Part model, mm, in its own coordinate system. A direction names the side the tool comes from. Give positions to 0.01 mm unless a question says otherwise; leave off trailing zeros. Write each loop counter-clockwise with the first axis right and the second up, starting at its lowest first coordinate (ties: lowest second). Pieces come first, ordered by that corner, then holes. Notation, with made-up numbers: M 56,62.5 L 106,62.5 A25 cw 106,94.5 Z; hole C 74,81 d3. An arc over 180 degrees is marked long. Answer as CSV lines item,"result". Start each with the question number.
Item 1: 3-axis set-ups, long thin cutter, end or side, ignore diameter. For faces 1 (the flat face through (99, -45, 9.669)), 2 (the flat face through (0, -41.5, 94)), 3 (the flat face through (0, -48.5, 94)), 4 (the flat face through (-91.805, -45, -10)), 5 (the flat face through (-99, -45, 9.669)): which of +Z, -Z, +X, -X, +Y, -Y reach the whole face in a straight line?
Item 2: Band-saw the part on A-A, the plane y = -32.25. List the corners of the cut face in (x, z) (3 decimals).
Item 3: Two-plate mould, pull along Y, no slides. Class faces 6 (the flat face through (91.805, -45, -10)), 7 (the cylindrical face through (99.41, -39.554, -7.481)), 8 (the flat face through (-99, -60, -6)): +Y half, -Y half, draft (parallel to the pull), parting line (faces both ways), or undercut.
Item 4: Wall check: L1, parallel to X at y = -46.5, z = 1 (3 decimals); L2, parallel to Z at x = -95.5, y = -40.25; L3, parallel to Y at x = -62.5, z = 73.5. Give the ranges that are in metal, low to high. Write a range as from..to.
Item 5: Band-saw the part on C-C, the plane z = 32. List the corners of the cut face in (x, y), then the cut area to 3 significant figures.
Item 6: Band-saw the part on B-B, the plane z = 82.5. List the corners of the cut face in (x, y).
Item 7: Band-saw the part on D-D, the plane x = 0. List the corners of the cut face in (y, z) (3 decimals), then the cut area to 3 significant figures.
Item 8: Pin check, flat tips, straight feed: pin 1 (4 mm diameter, centred on x = -47.5, y = -42, fed in from +Z); pin 2 (13 mm diameter, centred on y = -42.93, z = -5.33, fed in from -X) (3 decimals); pin 3 (4.5 mm diameter, centred on x = -100.5, y = -40.5, fed in from +Z); pin 4 (8 mm diameter, centred on x = -42.5, y = -46.5, fed in from -Z). Stop position of each tip, or through.
from build123d import *

# Parameters (mm, degrees)
BOSS_EXTRUDE1_DEPTH      = 60
CUT_EXTRUDE19_DEPTH      = 171.881965709
CUT_EXTRUDE19_DEPTH_BACK = 171.881965709
SKETCH30_W               = 213.61
SKETCH30_H               = 30
SKETCH31_R               = 4
CUT_EXTRUDE20_DEPTH      = 243.881988062
CUT_EXTRUDE21_DEPTH      = 11.5
CUT_EXTRUDE22_START      = -11.5
CUT_EXTRUDE22_DEPTH      = 11.5


with BuildPart() as part:
    # Sketch1 → Boss-Extrude1 (new body)
    with BuildSketch(Plane(origin=(0, 0, 0), x_dir=(1, 0, 0), z_dir=(0, 1, 0))):
        with BuildLine():
            Line((106.805, -9.669202779), (98.330740578, -9.669202779))
            ThreePointArc((98.330740578, -9.669202779), (0, -98.805), (-98.330740578, -9.669202779))
            Line((-98.330740578, -9.669202779), (-106.805, -9.669202779))
            Line((-106.805, -9.669202779), (-106.805, 20.330797221))
            Line((-106.805, 20.330797221), (-91.805, 20.330797221))
            Line((-91.805, 20.330797221), (-91.805, 0))
            ThreePointArc((-91.805, 0), (0, -91.805), (91.805, 0))
            Line((91.805, 0), (91.805, 20.330797221))
            Line((91.805, 20.330797221), (106.805, 20.330797221))
            Line((106.805, 20.330797221), (106.805, -9.669202779))
        make_face()
    extrude(amount=-BOSS_EXTRUDE1_DEPTH)

    # Sketch30 → Cut-Extrude19 (cut, two sides: drawn at the far end of the back side and taken through both)
    with BuildSketch(Plane(origin=(0, 0, -20.330797221), x_dir=(-1, 0, 0), z_dir=(0, 0, -1)).offset(-CUT_EXTRUDE19_DEPTH_BACK)):
        with Locations((0, -15)):
            Rectangle(SKETCH30_W, SKETCH30_H)
    extrude(amount=CUT_EXTRUDE19_DEPTH + CUT_EXTRUDE19_DEPTH_BACK, mode=Mode.SUBTRACT)

    # Sketch31 → Cut-Extrude20 (cut, through all)
    with BuildSketch(Plane(origin=(106.805, 0, 0), x_dir=(0, 0, -1), z_dir=(1, 0, 0))):
        with Locations((5.330797221, -42.92674227)):
            Circle(SKETCH31_R)
    extrude(amount=-CUT_EXTRUDE20_DEPTH, mode=Mode.SUBTRACT)

    # Sketch32 → Cut-Extrude21 (cut)
    with BuildSketch(Plane(origin=(0, -30, 0), x_dir=(1, 0, 0), z_dir=(0, 1, 0))):
        with BuildLine():
            Line((98.330740578, -9.669202779), (-98.330740578, -9.669202779))
            ThreePointArc((-98.330740578, -9.669202779), (0, -98.805), (98.330740578, -9.669202779))
        make_face()
    extrude(amount=-CUT_EXTRUDE21_DEPTH, mode=Mode.SUBTRACT)

    # Sketch33 → Cut-Extrude22 (cut)
    with BuildSketch(Plane(origin=(0, -60, 0), x_dir=(-1, 0, 0), z_dir=(0, -1, 0)).offset(CUT_EXTRUDE22_START)):
        with BuildLine():
            Line((98.330740578, -9.669202779), (-98.330740578, -9.669202779))
            ThreePointArc((-98.330740578, -9.669202779), (0, -98.805), (98.330740578, -9.669202779))
        make_face()
    extrude(amount=CUT_EXTRUDE22_DEPTH, mode=Mode.SUBTRACT)


solid = part.part
Output:
1,face 1,"+Z, +X"
1,face 2,"+Z, +X, -X, +Y"
1,face 3,"+Z, +X, -X, -Y"
1,face 4,"-Z, +Y, -Y"
1,face 5,"+Z, -X"
2,outline,"M -106.805,-20.331 L -91.805,-20.331 L -91.805,0 A91.805 cw -91.294,9.669 L -106.805,9.669 Z; M 91.294,9.669 A91.805 cw 91.805,0 L 91.805,-20.331 L 106.805,-20.331 L 106.805,9.669 Z"
3,face 6,"draft"
3,face 7,"undercut"
3,face 8,"-Y half"
4,L1,"-106.805..-91.8, 91.8..106.805"
4,L2,"-20.33..-8.3, -2.36..9.67"
4,L3,"-48.5..-41.5"
5,outline,"M -93.48,-48.5 L -86.05,-48.5 L -86.05,-41.5 L -93.48,-41.5 Z; M 86.05,-48.5 L 93.48,-48.5 L 93.48,-41.5 L 86.05,-41.5 Z"
5,area,"104 mm²"
6,outline,"M -54.37,-48.5 L -40.27,-48.5 L -40.27,-41.5 L -54.37,-41.5 Z; M 40.27,-48.5 L 54.37,-48.5 L 54.37,-41.5 L 40.27,-41.5 Z"
7,outline,"M -48.5,91.805 L -41.5,91.805 L -41.5,98.805 L -48.5,98.805 Z"
7,area,"49.0 mm²"
8,pin 1,"z = 87.71"
8,pin 2,"x = -106.805"
8,pin 3,"z = 9.67"
8,pin 4,"z = 79.16"
